from build123d import *

# Parameters (mm, degrees)
F1_DEPTH = 128
F2_R     = 2
F3_DEPTH = 25


with BuildPart() as f1:
    # F0 (on Top) → F1 (new body)
    with BuildSketch(Plane.XY):
        Polygon((12, -4), (12, 4), (-12, 4), (-12, -4), (-2, -4), (-2, 2), (2, 2), (2, -4), align=None)
    extrude(amount=F1_DEPTH)

    # F2 (on face) → F3 (cut)
    with BuildSketch(Plane(origin=(0, 4, 0), x_dir=(-1, 0, 0), z_dir=(0, 1, 0))):
        with Locations((-8, 8)):
            Circle(F2_R)
        with Locations((-8, 24)):
            Circle(F2_R)
        with Locations((-8, 40)):
            Circle(F2_R)
        with Locations((-8, 56)):
            Circle(F2_R)
        with Locations((-8, 72)):
            Circle(F2_R)
        with Locations((8, 8)):
            Circle(F2_R)
        with Locations((8, 24)):
            Circle(F2_R)
        with Locations((8, 40)):
            Circle(F2_R)
        with Locations((8, 56)):
            Circle(F2_R)
        with Locations((8, 72)):
            Circle(F2_R)
        with Locations((-8, 88)):
            Circle(F2_R)
        with Locations((-8, 104)):
            Circle(F2_R)
        with Locations((-8, 120)):
            Circle(F2_R)
        with Locations((8, 88)):
            Circle(F2_R)
        with Locations((8, 104)):
            Circle(F2_R)
        with Locations((8, 120)):
            Circle(F2_R)
    extrude(amount=-F3_DEPTH, mode=Mode.SUBTRACT)


solid = f1.part
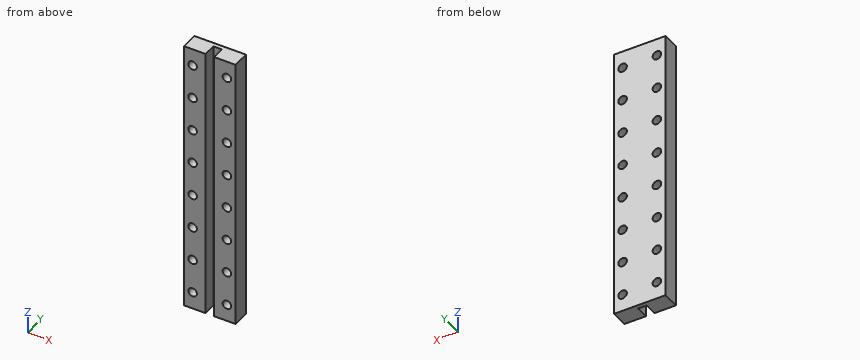
Source: CAD feature listing. Evaluate the final solid. Frame: model axes, mm. Coordinates: 2 decimals unless noted, no trailing zeros. Loops run counter-clockwise (first coordinate to the right, second up) from the corner with the lowest first, then second, coordinate; pieces in that order, holes last. Notation, with made-up numbers: (36, 72) - (87, 72) arc R26 ccw to (87, 95) - close; hole circle Ø9 at (58, -32). An arc over 180 degrees is marked (long way). Return JSON: item names as keys, results as strings.
Q1. Section A-A, the plane y = -0.5. Give the number of separate pieces and of enclosed holes in the cut face, plus the area to 3 significant figures.
Results:
{"separate pieces": "2", "enclosed holes": "16", "area": "2,360 mm2"}
Q2. Section B-B, the plane z = 72. Return loops of the section in (x, y).
Results:
{"outline": "(-12, -4) - (-10, -4) - (-10, 4) - (-12, 4) - close; (-6, -4) - (-2, -4) - (-2, 2) - (2, 2) - (2, -4) - (6, -4) - (6, 4) - (-6, 4) - close; (10, -4) - (12, -4) - (12, 4) - (10, 4) - close"}
Q3. Section D-D, the plane z = 15.5. Return loops of the section in (x, y).
Results:
{"outline": "(-12, -4) - (-2, -4) - (-2, 2) - (2, 2) - (2, -4) - (12, -4) - (12, 4) - (-12, 4) - close"}
Q4. Material intervals for line 1 along X through (y, z) = (1.25, 78); line 2 along Y through (x, z) = (-1.5, 43), sorted ascending.
Results:
{"line 1": "-12 to -2, 2 to 12", "line 2": "2 to 4"}
Q5. Contact query for flat-ended pins moving along their axis: P1, Ø3, axis at x = -1.5, y = 1, coming from the -Z side; P2, Ø2.5, axis at x = 8, z = 40, coming from the +Y side. Output: stop coordinate, or through.
Results:
{"P1": "z = 0", "P2": "through"}
